Geometry check sheet. Reference: the model listing, model coordinates, mm. A direction names the side the tool comes from. Round coordinates to 2 decimals unless told otherwise and drop trailing zeros. Order: outer loops, then holes, each group sorted by start corner. A loop starts at its lowest first (then second) coordinate and runs counter-clockwise, first axis right, second up.
```python
from build123d import *

# Parameters (mm, degrees)
SKETCH1_R           = 1.75
BOSS_EXTRUDE1_DEPTH = 6


with BuildPart() as part:
    # Sketch1 → Boss-Extrude1 (new body)
    with BuildSketch(Plane(origin=(0, 0, 0), x_dir=(1, 0, 0), z_dir=(0, 1, 0))):
        with BuildLine():
            Line((-56.568542495, -15), (-116.568542495, -15))
            ThreePointArc((-116.568542495, -15), (-120.104076401, -16.464466094), (-121.568542495, -20))
            Line((-121.568542495, -20), (-121.568542495, -90))
            ThreePointArc((-121.568542495, -90), (-123.033008589, -93.535533906), (-126.568542495, -95))
            Line((-126.568542495, -95), (-256.568542495, -95))
            ThreePointArc((-256.568542495, -95), (-260.104076401, -93.535533906), (-261.568542495, -90))
            Line((-261.568542495, -90), (-261.568542495, 90))
            ThreePointArc((-261.568542495, 90), (-260.104076401, 93.535533906), (-256.568542495, 95))
            Line((-256.568542495, 95), (-126.568542495, 95))
            ThreePointArc((-126.568542495, 95), (-123.033008589, 93.535533906), (-121.568542495, 90))
            Line((-121.568542495, 90), (-121.568542495, 20))
            ThreePointArc((-121.568542495, 20), (-120.104076401, 16.464466094), (-116.568542495, 15))
            Line((-116.568542495, 15), (-56.568542495, 15))
            ThreePointArc((-56.568542495, 15), (-53.681791149, 15.917517095), (-51.854497287, 18.333333333))
            ThreePointArc((-51.854497287, 18.333333333), (55, 0), (-51.854497287, -18.333333333))
            ThreePointArc((-51.854497287, -18.333333333), (-53.681791149, -15.917517095), (-56.568542495, -15))
        make_face()
        with Locations(Location((31.851272196, -31.788306962, 0), (0, 0, 270))):
            Circle(SKETCH1_R, mode=Mode.SUBTRACT)
        with Locations(Location((31.788306962, 31.851272196, 0), (0, 0, 270))):
            Circle(SKETCH1_R, mode=Mode.SUBTRACT)
        with Locations(Location((-31.851272196, 31.788306962, 0), (0, 0, 270))):
            Circle(SKETCH1_R, mode=Mode.SUBTRACT)
        with Locations(Location((-31.788306962, -31.851272196, 0), (0, 0, 270))):
            Circle(SKETCH1_R, mode=Mode.SUBTRACT)
    extrude(amount=BOSS_EXTRUDE1_DEPTH)


solid = part.part
```
(1) Depth check by flat-ended pin: P1, Ø2, axis at x = -74, y = 4, coming from the -Z side; P2, Ø4, axis at x = 31.79, z = -31.85, coming from the -Y side; P3, Ø1, axis at y = 3, z = 24.5, coming from the +X side. Enter the tip coordinate at first touch or a pass-through.
Returned:
P1: stops at z = -15
P2: stops at y = 0
P3: stops at x = 49.49
(2) Sectioned sample at C-C, the plane y = 2.5. Record the cut outline in (x, z).
Returned:
outline: (-261.57, -90) arc R5 ccw to (-256.57, -95) - (-126.57, -95) arc R5 ccw to (-121.57, -90) - (-121.57, -20) arc R5 cw to (-116.57, -15) - (-56.57, -15) arc R5 cw to (-51.85, -18.33) arc R55 ccw (long way) to (-51.85, 18.33) arc R5 cw to (-56.57, 15) - (-116.57, 15) arc R5 cw to (-121.57, 20) - (-121.57, 90) arc R5 ccw to (-126.57, 95) - (-256.57, 95) arc R5 ccw to (-261.57, 90) - close; hole circle Ø3.5 at (-31.85, -31.79); hole circle Ø3.5 at (-31.79, 31.85); hole circle Ø3.5 at (31.79, -31.85); hole circle Ø3.5 at (31.85, 31.79)
(3) Draft check along X on faces 4 (the flat face through (-192, 3, -95)), 5 (the flat face through (-87, 3, -15)), 6 (the flat face through (-261.569, 3, 1)). Enter one of: released by +X, released by -X, zero draft, split by the parting line, or undercut.
Returned:
face 4: zero draft
face 5: undercut
face 6: released by -X
(4) Set-up check for faces 1 (the flat face through (-121.569, 3, -55)), 2 (the flat face through (-121.569, 3, 55)), 3 (the cylindrical face through (54.958, 2.958, -2.157)): record each of +Z, -Z, +X, -X, +Y, -Y from which the full face is reachable in a straight line by a thin tool's end or side.
Returned:
face 1: -Z, +Y, -Y
face 2: +Z, +Y, -Y
face 3: +Y, -Y
(5) Material ranges on line 1 (X direction, y = 1.85, z = 20.5); line 2 (X direction, y = 4.85, z = 70.5); line 3 (Z direction, x = -59, y = 2.55), recorded low to high.
Returned:
line 1: x = -261.57 to -121.57, -51.04 to 51.04
line 2: x = -261.57 to -121.57
line 3: z = -15 to 15
(6) Sectioned sample at D-D, the plane z = 51. Record the cut outline in (x, y).
Returned:
outline: (-261.57, 0) - (-121.57, 0) - (-121.57, 6) - (-261.57, 6) - close; (-20.59, 0) - (20.59, 0) - (20.59, 6) - (-20.59, 6) - close
(7) Sectioned sample at A-A, the plane z = -50.5. Record the cut outline in (x, y).
Returned:
outline: (-261.57, 0) - (-121.57, 0) - (-121.57, 6) - (-261.57, 6) - close; (-21.79, 0) - (21.79, 0) - (21.79, 6) - (-21.79, 6) - close
(8) Sectioned sample at B-B, the plane x = 0. Record the cut outline in (y, z), and give its area (3 significant figures).
Returned:
outline: (0, -55) - (6, -55) - (6, 55) - (0, 55) - close
area: 660 mm2
